The listing builds one solid part. Answer for the finished solid, in the listing's coordinates (mm). Give positions to 0.01 mm unless a question says otherwise; leave off trailing zeros. Loops run counter-clockwise (first coordinate to the right, second up) from the corner with the lowest first, then second, coordinate; pieces in that order, holes last. Notation, with made-up numbers: (72.25, -6) - (130.25, -6) arc R27 ccw to (130.25, 15) - close; hole circle Ø2 at (68, 58.5). An arc over 180 degrees is marked (long way). One line per item, written item: value. Start each with the question number.
from build123d import *

# Parameters (mm, degrees)
SKETCH2_W           = 50
SKETCH2_H           = 100
BOSS_EXTRUDE1_DEPTH = 150
CUT_EXTRUDE1_DEPTH  = 150


with BuildPart() as part:
    # Sketch2 → Boss-Extrude1 (new body)
    with BuildSketch(Plane.XY):
        Rectangle(SKETCH2_W, SKETCH2_H)
    extrude(amount=BOSS_EXTRUDE1_DEPTH)

    # Sketch3 → Cut-Extrude1 (cut)
    with BuildSketch(Plane.ZY.offset(25)):
        Polygon((150, 0), (100, -50), (150, -50), align=None)
    extrude(amount=-CUT_EXTRUDE1_DEPTH, mode=Mode.SUBTRACT)


solid = part.part
1. Find the intervals of material crossed by L1, parallel to Z at x = 7.5, y = -8; L2, parallel to Y at x = 5, z = 141.5; L3, parallel to Y at x = 16.5, z = 106, in increasing order. Write a range as [from, to].
2. A cutting plane is placed at A-A (x = -12.5). Determine the outline of the cut face in (y, z).
3. A cutting plane is placed at B-B (z = 102). Determine the outline of the cut face in (x, y).
Results below:
1. L1: z = [0, 142]
1. L2: y = [-8.5, 50]
1. L3: y = [-44, 50]
2. outline: (-50, 0) - (50, 0) - (50, 150) - (0, 150) - (-50, 100) - close
3. outline: (-25, -48) - (25, -48) - (25, 50) - (-25, 50) - close
